Geometry: final body of the model. Coordinates: model frame, mm. Give positions to 0.01 mm unless a question says otherwise; leave off trailing zeros. Write each loop counter-clockwise with the first axis right and the second up, starting at its lowest first coordinate (ties: lowest second). Pieces come first, ordered by that corner, then holes. Notation, with made-up numbers: (5, -35.5) -> (34, -35.5) arc R25 cw to (34, -1.5) -> close; hole circle Ø2 at (77.5, 67.25). An arc over 180 degrees is marked (long way). Answer in a Markdown table with one row per item. Add a question column.
Item 1: Section query B-B on x = -3.75. Output: boundary loops of the cut face in (y, z).
Item 2: First-contact query: P1, Ø0.8, axis at x = -0.5, z = 287, coming from the +Y side; P2, Ø1.1, axis at x = -0.5, z = 310.5, coming from the -Y side; P3, Ø4.5, axis at x = -4, z = 119.5, coming from the +Y side; P4, Ø1.5, axis at x = -3.5, y = -6, coming from the -Z side. Flat tips, straight axial feed; report the tip coordinate or a pass-through.
Item 3: Section query A-A on z = 138. Output: boundary loops of the cut face in (x, y), plus the area to 3 significant figures.
Item 4: Draft query along Y for faces 1 (the flat face through (-1, 2, 221)), 2 (the flat face through (-0.7, -1.2, 449.262)). Return one class per face: +Y half, -Y half, draft (parallel to the pull), parting line (faces both ways), or undercut.
Item 5: Material intervals for probe 1 along Y at (x, z) = (-2.5, 160); probe 2 along Y at (x, z) = (-1.25, 180); probe 3 along X at (y, z) = (6.5, 150), sorted ascending. Write a range as from..to.
Item 6: Section query C-C on y = -7.5. Output: boundary loops of the cut face in (x, z).
```python
from build123d import *

# Parameters (mm, degrees)
EXTRUDE_THIN1_DEPTH = 449.2625
CUT_EXTRUDE1_START  = -8.5
CUT_EXTRUDE1_DEPTH  = 9.5
LPATTERN1_COUNT     = 18
LPATTERN1_PITCH     = 25
FILLET1_R           = 0.5


with BuildPart() as part:
    # Sketch3 → Extrude-Thin1 (new body)
    with BuildSketch(Plane.XY):
        Polygon((-6.5, 17.5), (-6.5, 13.5), (0, 13.5), (0, -13.5), (-6.5, -13.5), (-6.5, -17.5), (-7.5, -17.5), (-7.5, -12.5), (-1, -12.5), (-1, 12.5), (-7.5, 12.5), (-7.5, 17.5), align=None)
    extrude(amount=EXTRUDE_THIN1_DEPTH)

    # Sketch4 → Cut-Extrude1 (cut)
    with BuildSketch(Plane(origin=(0, 0, 0), x_dir=(0, 0, -1), z_dir=(1, 0, 0)).offset(CUT_EXTRUDE1_START)):
        with BuildLine():
            Line((-6.65, -3.15), (-18.35, -3.15))
            ThreePointArc((-18.35, -3.15), (-21.5, 0), (-18.35, 3.15))
            Line((-18.35, 3.15), (-6.65, 3.15))
            ThreePointArc((-6.65, 3.15), (-3.5, 0), (-6.65, -3.15))
        make_face()
    cut_extrude1 = extrude(amount=CUT_EXTRUDE1_DEPTH, mode=Mode.SUBTRACT)

    # LPattern1: Cut-Extrude1 ×18
    with Locations(*[(0, 0, i * LPATTERN1_PITCH) for i in range(1, LPATTERN1_COUNT)]):
        add(cut_extrude1, mode=Mode.SUBTRACT)

    # Fillet1
    fillet1_edges = [part.edges().sort_by_distance(p)[0] for p in [
        (-6.5, 13.5, 224.63125),
        (0, 13.5, 224.63125),
        (0, -13.5, 224.63125),
        (-6.5, -13.5, 224.63125),
        (-7.5, -12.5, 224.63125),
        (-1, -12.5, 224.63125),
        (-1, 12.5, 224.63125),
        (-7.5, 12.5, 224.63125),
    ]]
    fillet(fillet1_edges, radius=FILLET1_R)


solid = part.part
```
Findings below:
| question | item | result |
|---|---|---|
| 1 | outline | (-13.5, 0) -> (-12.5, 0) -> (-12.5, 449.26) -> (-13.5, 449.26) -> close; (12.5, 0) -> (13.5, 0) -> (13.5, 449.26) -> (12.5, 449.26) -> close |
| 2 | P1 | stops at y = 13.5 |
| 2 | P2 | stops at y = -13.5 |
| 2 | P3 | stops at y = 13.57 |
| 2 | P4 | passes through |
| 3 | outline | (-7.5, -17.5) -> (-6.5, -17.5) -> (-6.5, -14) arc R0.5 cw to (-6, -13.5) -> (-0.5, -13.5) arc R0.5 ccw to (0, -13) -> (0, -3.15) -> (-1, -3.15) -> (-1, -12) arc R0.5 cw to (-1.5, -12.5) -> (-7, -12.5) arc R0.5 ccw to (-7.5, -13) -> close; (-7.5, 13) arc R0.5 ccw to (-7, 12.5) -> (-1.5, 12.5) arc R0.5 cw to (-1, 12) -> (-1, 3.15) -> (0, 3.15) -> (0, 13) arc R0.5 ccw to (-0.5, 13.5) -> (-6, 13.5) arc R0.5 cw to (-6.5, 14) -> (-6.5, 17.5) -> (-7.5, 17.5) -> close |
| 3 | area | 41.7 mm^2 |
| 4 | face 1 | undercut |
| 4 | face 2 | draft |
| 5 | probe 1 | y = -13.5..-12.5, 12.5..13.5 |
| 5 | probe 2 | y = -13.5..-12.43, 12.43..13.5 |
| 5 | probe 3 | x = -1..0 |
| 6 | outline | (-1, 0) -> (0, 0) -> (0, 449.26) -> (-1, 449.26) -> close |
